Here's how the part is built. I have some questions about the finished solid (model axes, mm). Coordinates: 2 decimals unless noted, no trailing zeros. Order: outer loops, then holes, each group sorted by start corner. A loop starts at its lowest first (then second) coordinate and runs counter-clockwise, first axis right, second up. Notation, with made-up numbers: (26, 73.5) - (81, 73.5) arc R31 cw to (81, 107.5) - close; hole circle Ø9 at (89, 57.25). An arc over 180 degrees is marked (long way). Answer in a Markdown table with one row per item. Add a question column.
Item 1: Will these pins go through, and if not, where does the flat tip stop? pin 1 Ø8 at (x, z) = (-5.5, 5) entering from +Y; pin 2 Ø10 at (x, y) = (-89, 7) entering from -Z; pin 3 Ø12 at (x, z) = (89.5, -11.5) entering from +Y.
Item 2: I want a section at A-A (x = -9.5). Please give me the cut outline in (y, z).
Item 3: I want a section at B-B (x = -85). Please give me the cut outline in (y, z), plus the area to 3 significant figures.
Item 4: If I drill on line 1 along X through (y, z) = (17.5, -16); line 2 along X through (y, z) = (-3, 10); line 3 along Z through (x, y) = (165, 13.5), over which ranges is the centre line in solid material (lowest first)? Write a range as from..to.
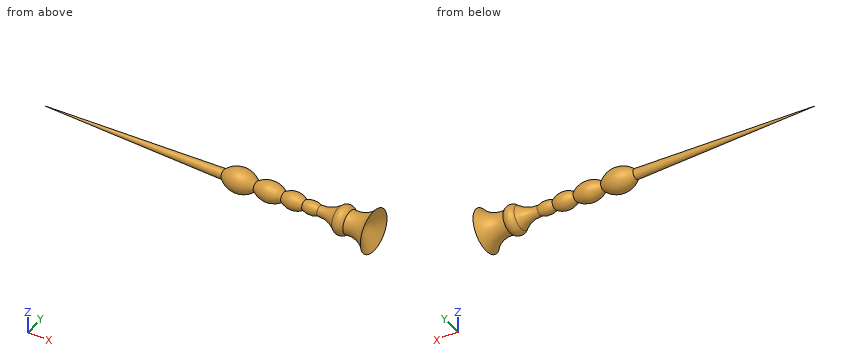
```python
from build123d import *


with BuildPart() as f1:
    # F0 (on Top) → F1 (revolve)
    with BuildSketch(Plane.XY):
        with BuildLine():
            Line((40.465098, 17.228693), (-147.924334, 12.066938))
            Line((-147.924334, 12.066938), (182.042071, 12.066938))
            Line((182.042071, 12.066938), (196.13757, 34.00075))
            ThreePointArc((196.13757, 34.00075), (185.195735, 25.646108), (171.541095, 23.892656))
            ThreePointArc((171.541095, 23.892656), (165.739328, 26.680922), (159.937561, 23.892656))
            ThreePointArc((159.937561, 23.892656), (150.673117, 18.605893), (140.095636, 17.228693))
            ThreePointArc((140.095636, 17.228693), (132.277064, 18.842771), (124.458492, 17.228693))
            ThreePointArc((124.458492, 17.228693), (113.572422, 20.759941), (102.686353, 17.228693))
            ThreePointArc((102.686353, 17.228693), (88.368863, 22.224471), (74.051373, 17.228693))
            ThreePointArc((74.051373, 17.228693), (57.258235, 24.209892), (40.465098, 17.228693))
        make_face()
    revolve(axis=Axis((13.855253, 12.066938, 0), (1, 0, 0)))


solid = f1.part
```
Values follow:
| question | item | result |
|---|---|---|
| 1 | pin 1 | stops at y = 15.84 |
| 1 | pin 2 | stops at z = -1.63 |
| 1 | pin 3 | stops at y = 20.58 |
| 2 | outline | circle Ø7.59 at (12.07, 0) |
| 3 | outline | circle Ø3.45 at (12.07, 0) |
| 3 | area | 9.34 mm^2 |
| 4 | line 1 | x = 191.04..192.9 |
| 4 | line 2 | x = 192.5..193.66 |
| 4 | line 3 | z = -14.51..14.51 |
